Autodesk Inventor part; units mm, degrees
ref_plane "YZ Plane" through (0, 0, 0) normal (1, 0, 0) x (0, 1, 0)
ref_plane "XZ Plane" through (0, 0, 0) normal (0, 1, 0) x (-1, 0, 0)
ref_plane "XY Plane" through (0, 0, 0) normal (0, 0, 1) x (1, 0, 0)
sketch "Sketch1" plane through (0, 0, 0) normal (0, 0, 1) x (1, 0, 0)
  circle A0 centre (0, 0) radius 10
  line L0 (0, 10) -> (30, 10)
  arc A1 (0, -10) -> (30, 10) centre (6.2119, 13.1822) ccw
  circle A2 centre (0, 0) radius 3.5
  circle A3 centre (0, 0) radius 7.5
  circle A4 centre (0, 0) radius 6
  dimension "d0" = 20
  dimension "d1" = 30
  dimension "d2" = 24
  dimension "d3" = 10
  dimension "d4" = 13.1822
  dimension "d5" = 7
  dimension "d6" = 15
  dimension "d7" = 12
extrude "Extrusion1" add sketch "Sketch1" along normal mid plane 20 contours A0 L0 A1
extrude "Extrusion2" add sketch "Sketch1" along normal mid plane 4 contours A0 | A3 | A4
extrude "Extrusion3" add sketch "Sketch1" along normal mid plane 8 contours A3 | A4
extrude "Extrusion4" add sketch "Sketch1" along normal mid plane 12 contours A4
sketch "Sketch2" plane through (0, 0, 6) normal (0, 0, 1) x (1, 0, 0)
  circle A0 centre (0, 0) radius 7.5
  circle A1 centre (0, 0) radius 3.5
  dimension "d16" = 15
  dimension "d18" = 7
sketch "Sketch3" plane through (0, 0, -6) normal (0, 0, -1) x (-1, 0, 0)
  circle A0 centre (0, 0) radius 7.5
  circle A1 centre (0, 0) radius 3.5
  dimension "d17" = 15
  dimension "d19" = 7
extrude "Extrusion5" add sketch "Sketch3" along normal blind 2
extrude "Extrusion6" add sketch "Sketch2" along normal blind 2
fillet "Fillet1" radius 4 4 edges at (15, 10, -10) (19.5247, -6.7871, -10) (19.5247, -6.7871, 10) (15, 10, 10)
properties part number "TapPart"
CAD build for the part. Positions are in the model's coordinates, mm. A direction names the side the tool comes from. Round coordinates to 2 decimals unless told otherwise and drop trailing zeros. Order: outer loops, then holes, each group sorted by start corner. A loop starts at its lowest first (then second) coordinate and runs counter-clockwise, first axis right, second up. Notation, with made-up numbers: (-0.5, 85) -> (37.5, 85) arc R17 cw to (37.5, 104) -> close; hole circle Ø6 at (1.25, 4). An arc over 180 degrees is marked (long way). Write item = value, one per line.
(1) Flat gauge pins, fed straight in: P1, Ø2, axis at y = 5, z = 4, coming from the +X side; P2, Ø4.5, axis at x = 1.5, y = -3.5, coming from the +Z side; P3, Ø12, axis at x = -3.5, y = -1, coming from the -Z side; P4, Ø10, axis at x = 4.5, y = -3.5, coming from the +Z side. Where does each tip first touch, or does it go through?
Answers follow:
P1 = 29.11
P2 = 8
P3 = -8
P4 = 10
(2) Cut at C-C (z = 5). Write the cut outline in (x, y), plus the area to 3 significant figures.
Answers follow:
outline = circle Ø12 at (0, 0); (0, -10) arc R24 ccw to (30, 10) -> (0, 10) arc R10 cw to start; hole circle Ø7 at (0, 0)
area = 421 mm²
(3) Cut at A-A (z = 2.75). Write the cut outline in (x, y), plus the area to 3 significant figures.
Answers follow:
outline = circle Ø15 at (0, 0); (0, -10) arc R24 ccw to (30, 10) -> (0, 10) arc R10 cw to start; hole circle Ø7 at (0, 0)
area = 485 mm²
(4) Pull direction Z, two halves, no side cores. Call faces 1 (the cylindrical face through (14.79, 8.797, 8.859)), 2 (the cylindrical face through (-6, 0, -5)), 3 (the cylindrical face through (-10, 0, 0)): +Z half, -Z half, draft (parallel to the pull), parting line (faces both ways), or undercut.
Answers follow:
face_1 = +Z half
face_2 = undercut
face_3 = draft
(5) Drill centre lines: L1, parallel to Z at x = -6.5, y = -3.5; L2, parallel to Y at x = 0, z = -1.75; L3, parallel to X at y = 2.25, z = -6.5. Where is each one in solid material? Low to high.
Answers follow:
L1 = -8 to -6, -4 to 4, 6 to 8
L2 = -10 to -3.5, 3.5 to 10
L3 = -7.15 to -2.68, 2.68 to 7.15, 9.74 to 27.54
(6) 3-axis set-ups, long thin cutter, end or side, ignore diameter. For faces 4 (the cylindrical face through (-7.493, 0.33, 3.014)), 5 (the flat face through (4, 7, -2)), 6 (the flat face through (2, 6, -4)): which of +Z, -Z, +X, -X, +Y, -Y reach the whole face in a straight line?
Answers follow:
face_4 = +Z
face_5 = -Z
face_6 = none
